```python
from build123d import *

# Parameters (mm, degrees)
F0_W      = 104
F0_H      = 60
F0_W_2    = 85
F0_H_2    = 56
F1_DEPTH  = 8.5
F2_DEPTH  = 2
F3_W      = 8.5
F3_H      = 3
F4_DEPTH  = 2.5
F5_SIZE   = 1
F6_DEPTH  = 5
F7_W      = 5
F7_H      = 10
F8_DEPTH  = 8
F9_W      = 5
F9_H      = 60
F10_DEPTH = 5.5


with BuildPart() as f1:
    # F0 (on Top) → F1 (new body)
    with BuildSketch(Plane.XY):
        with Locations((1.1924776137, -7.5798341542)):
            Rectangle(F0_W, F0_H)
        with Locations((-0.8075223863, -7.5798341542)):
            Rectangle(F0_W_2, F0_H_2, mode=Mode.SUBTRACT)
    extrude(amount=F1_DEPTH)

    # F0 (on Top) → F2 (join)
    with BuildSketch(Plane.XY):
        with Locations((-0.8075223863, -7.5798341542)):
            Rectangle(F0_W_2, F0_H_2)
        Polygon((-35.8075223863, -32.5798341542), (-35.8075223863, 17.4201658458), (34.1924776137, 17.4201658458), (38.1924776137, 17.4201658458), (38.1924776137, -32.5798341542), align=None, mode=Mode.SUBTRACT)
    extrude(amount=F2_DEPTH)

    # F3 (on face) → F4 (join)
    with BuildSketch(Plane.XY.offset(8.5)):
        with Locations((37.4424776137, -34.0798341542)):
            Rectangle(F3_W, F3_H)
        with Locations((37.4424776137, 18.9201658458)):
            Rectangle(F3_W, F3_H)
        Polygon((33.1924776137, -37.5798341542), (53.1924776137, -37.5798341542), (53.1924776137, -32.5798341542), (41.6924776137, -32.5798341542), (41.6924776137, -35.5798341542), (33.1924776137, -35.5798341542), align=None)
        Polygon((41.6924776137, 17.4201658458), (53.1924776137, 17.4201658458), (53.1924776137, 22.4201658458), (33.1924776137, 22.4201658458), (33.1924776137, 20.4201658458), (41.6924776137, 20.4201658458), align=None)
    extrude(amount=F4_DEPTH)

    # F5
    f5_edges = [f1.edges().sort_by_distance(p)[0] for p in [
        (33.192478, 18.920166, 8.5),
        (33.192478, -34.079834, 8.5),
    ]]
    chamfer(f5_edges, length=F5_SIZE)

    # F6 (cut): a face of the model
    f6_faces = [f1.faces().sort_by_distance(p)[0] for p in [
        (47.4424776137, -7.5798341542, 8.5),
    ]]
    extrude(f6_faces, amount=-F6_DEPTH, mode=Mode.SUBTRACT)

    # F7 (on face) → F8 (join)
    with BuildSketch(Plane.XY.offset(11)):
        Polygon((53.1924776137, 17.4201658458), (53.1924776137, 12.4201658458), (58.1924776137, 12.4201658458), (58.1924776137, 22.4201658458), (53.1924776137, 22.4201658458), align=None)
        with Locations((55.6924776137, -32.5798341542)):
            Rectangle(F7_W, F7_H)
    extrude(amount=-F8_DEPTH)

    # F9 (on face) → F10 (join)
    with BuildSketch(Plane.XY.offset(8.5)):
        with Locations((-53.3075223863, -7.5798341542)):
            Rectangle(F9_W, F9_H)
    extrude(amount=-F10_DEPTH)


solid = f1.part
```
The listing builds one solid part. Answer for the finished solid, in the listing's coordinates (mm). A direction names the side the tool comes from. Give positions to 0.01 mm unless a question says otherwise; leave off trailing zeros. Write each loop counter-clockwise with the first axis right and the second up, starting at its lowest first coordinate (ties: lowest second). Pieces come first, ordered by that corner, then holes. Notation, with made-up numbers: M 52,31 L 91,31 A15 ccw 91,59 Z; hole C 57,75 d5. An arc over 180 degrees is marked long. Write each question's results on one line, items separated by ' | '.
Q1. For a pull along Y with two mould halves and no side action, classify faces 6 (the flat face through (-53, -7, 3)), 7 (the flat face through (56, -27.58, 7)) as released by +Y, released by -Y, zero draft, split by the parting line, or undercut.
Output values:
face 6: zero draft | face 7: undercut
Q2. Flat-ended cylindrical pins translate along their axes: P1, Ø4, axis at x = -53, y = 6, coming from the -Z side; P2, Ø1.8, axis at y = -16, z = 2.5, coming from the +X side; P3, Ø4, axis at x = -43.5, y = 3.5, coming from the +Z side. Find the tip coordinate at first contact, or state that the pin passes through.
Output values:
P1: z = 3 | P2: x = 53.19 | P3: z = 8.5
Q3. Section A-A, the plane y = 16 is taken. Write down the section's boundary in (x, z), then the cut area to 4 significant figures.
Output values:
outline: M -55.81,3 L -50.81,3 L -50.81,0 L -35.81,0 L -35.81,2 L -43.31,2 L -43.31,8.5 L -55.81,8.5 Z; M 38.19,0 L 53.19,0 L 53.19,3 L 58.19,3 L 58.19,11 L 53.19,11 L 53.19,3.5 L 41.69,3.5 L 41.69,2 L 38.19,2 Z | area: 193.5 mm2
Q4. Section B-B, the plane x = 35.5 is taken. Write down the section's boundary in (y, z).
Output values:
outline: M -37.58,0 L -32.58,0 L -32.58,2 L -35.58,2 L -35.58,8.5 L -32.58,8.5 L -32.58,11 L -37.58,11 Z; M 17.42,0 L 22.42,0 L 22.42,11 L 17.42,11 L 17.42,8.5 L 20.42,8.5 L 20.42,2 L 17.42,2 Z
Q5. Section D-D, the plane y = -21.5 is taken. Write down the section's boundary in (x, z), then the cut area to 4 significant figures.
Output values:
outline: M -55.81,3 L -50.81,3 L -50.81,0 L -35.81,0 L -35.81,2 L -43.31,2 L -43.31,8.5 L -55.81,8.5 Z; M 38.19,0 L 53.19,0 L 53.19,3.5 L 41.69,3.5 L 41.69,2 L 38.19,2 Z | area: 153.5 mm2
Q6. A tool of negligible diameter and unlimited length cuts with its end or side. For faces 1 (the flat face through (38, 19, 8.5)), 2 (the flat face through (-44, -7, 8.5)), 3 (the flat face through (46, -32.58, 8)), 4 (the flat face through (2, -32.58, 1)), 5 (the flat face through (56, 17, 3)), from which of +Z, -Z, +X, -X, +Y, -Y can it reach the whole face along a straight path? Write none if from no direction.
Output values:
face 1: none | face 2: +Z, -X, +Y, -Y | face 3: +Z | face 4: +Z, -Z | face 5: -Z, +X, +Y, -Y
Q7. Consider L1, parallel to Y at x = 16, z = 5.75; L2, parallel to Y at x = -16.5, z = 0.75; L3, parallel to Z at x = -36.5, y = -13.5. Determine where each line is inside the solid, lowest interval first. Write a range as from..to.
Output values:
L1: -37.58..-35.58, 20.42..22.42 | L2: -37.58..-32.58, 17.42..22.42 | L3: 0..2
Q8. Section C-C, the plane z = 5.5 is taken. Write down the section's boundary in (x, y), then the cut area to 4 significant figures.
Output values:
outline: M -55.81,-37.58 L 58.19,-37.58 L 58.19,-27.58 L 53.19,-27.58 L 53.19,-32.58 L 41.69,-32.58 L 41.69,-35.58 L -43.31,-35.58 L -43.31,20.42 L 41.69,20.42 L 41.69,17.42 L 53.19,17.42 L 53.19,12.42 L 58.19,12.42 L 58.19,22.42 L -55.81,22.42 Z | area: 1,305 mm2
